Can you work these out from the model? Positions are in its coordinate system, mm. Face numbers are marked on the shaded views. Give positions to 0.01 mm unless a question says otherwise; leave off trailing zeros. Write each loop counter-clockwise with the first axis right and the second up, starting at its lowest first coordinate (ties: lowest second). Pieces come first, ordered by that corner, then holes. Notation, with made-up numbers: (-32, 84.25) -> (-7, 84.25) arc R33 ccw to (-7, 114.25) -> close; hole circle Ø1 at (7.25, -38.5). An arc over 180 degrees is marked (long way). Answer as CSV lines item,"result". Start each with the question number.
1. I need wall thicknesses on line 1 (Y direction, x = 52.5, z = 0.55); line 2 (Y direction, x = -52.5, z = 1.25); line 3 (Y direction, x = 32.5, z = -1.75). Which ranges of each line are inside material? Lowest first, please. Write a range as [from, to].
2. If we section it at D-D on y = -25: Write out the boundary of the cut face in (x, z), plus the area to 3 significant figures.
3. If we section it at B-B on x = 0: Write out the boundary of the cut face in (y, z).
4. I'm going to push flat-ended pins straight in: P1, Ø1.1, axis at x = -16.5, z = -2, coming from the +Y side; P2, Ø9.5, axis at x = -13, y = 5, coming from the +Z side; P3, Ø2, axis at x = -28, z = -2, coming from the -Y side; P4, Ø5, axis at x = -18, y = 22.5, coming from the +Z side. Where does each tip first touch, or does it pass through?
5. If we mould it in two halves opening along Y, with no side actions, what happens to the marked faces 1 and 2? For each: pulls with the +Y half, pulls with the -Y half, needs draft (parallel to the pull), parting line crosses it, or undercut.
6. If we section it at C-C on z = 0.65: Count the separate pieces of the cut face and the enclosed holes in it, plus the area to 3 significant figures.
7. If we section it at A-A on x = -52.5: Write out the boundary of the cut face in (y, z).
```python
from build123d import *

# Parameters (mm, degrees)
SKETCH_1_W          = 113
SKETCH_1_H          = 37
SKETCH_1_R          = 2
EXTRUDE_1_DEPTH     = 2.5
SKETCH_2_W          = 12
SKETCH_2_H          = 15
CUT_EXTRUDE_1_DEPTH = 6
CUT_EXTRUDE_2_DEPTH = 1
FILLET_1_R          = 2
FILLET_2_R          = 2
EXTRUDE_2_DEPTH     = 5
FILLET_3_R          = 10
SKETCH_5_R          = 1.75
CUT_EXTRUDE_3_DEPTH = 6


with BuildPart() as part:
    # 草图1 → 凸台-拉伸1 (new body, symmetric)
    with BuildSketch(Plane.XY):
        Rectangle(SKETCH_1_W, SKETCH_1_H)
        with Locations((52.5, 14.5)):
            Circle(SKETCH_1_R, mode=Mode.SUBTRACT)
        with Locations((52.5, -14.5)):
            Circle(SKETCH_1_R, mode=Mode.SUBTRACT)
        with Locations((-52.5, -14.5)):
            Circle(SKETCH_1_R, mode=Mode.SUBTRACT)
        with Locations((-52.5, 14.5)):
            Circle(SKETCH_1_R, mode=Mode.SUBTRACT)
    extrude(amount=EXTRUDE_1_DEPTH, both=True)

    # 草图2 → 切除-拉伸1 (cut, through all)
    with BuildSketch(Plane(origin=(0, 0, -2.5), x_dir=(-1, 0, 0), z_dir=(0, 0, -1))):
        with Locations((50.5, 0)):
            Rectangle(SKETCH_2_W, SKETCH_2_H)
    extrude(amount=-CUT_EXTRUDE_1_DEPTH, mode=Mode.SUBTRACT)

    # 草图3 → 切除-拉伸2 (cut)
    with BuildSketch(Plane(origin=(0, 0, -2.5), x_dir=(-1, 0, 0), z_dir=(0, 0, -1))):
        Polygon((-48.5, -15.5), (48.500097741, -15.5), (48.500097741, -10.5), (41.5, -10.5), (41.5, 10.420732232), (48.500097741, 10.420732232), (48.526939222, 15.5), (-48.5, 15.5), align=None)
    cut_extrude_2 = extrude(amount=-CUT_EXTRUDE_2_DEPTH, mode=Mode.SUBTRACT)

    # 圆角1
    fillet_1_edges = [part.edges().sort_by_distance(p)[0] for p in [
        (48.5, -15.5, -2),
        (48.5, 15.5, -2),
        (-48.526939222, 15.5, -2),
        (-48.500097741, 10.420732232, -2),
        (-41.5, 10.420732232, -2),
        (-41.5, -10.5, -2),
        (-48.500097741, -10.5, -2),
        (-48.500097741, -15.5, -2),
    ]]
    fillet(fillet_1_edges, radius=FILLET_1_R)

    # 圆角2
    fillet_2_edges = [part.edges().sort_by_distance(p)[0] for p in [
        (-56.5, 7.5, 0),
        (-56.5, -7.5, 0),
        (-44.5, -7.5, 0),
        (-44.5, 7.5, 0),
        (-56.5, 18.5, 0),
        (56.5, 18.5, 0),
        (56.5, -18.5, 0),
        (-56.5, -18.5, 0),
    ]]
    fillet(fillet_2_edges, radius=FILLET_2_R)

    # 草图4 → 凸台-拉伸2 (add)
    with BuildSketch(Plane(origin=(0, 0, -2.5), x_dir=(-1, 0, 0), z_dir=(0, 0, -1))):
        Polygon((17.5, 18.5), (0, 33.5), (-17.5, 18.5), align=None)
        Polygon((17.5, -18.5), (-17.5, -18.5), (0, -33.5), align=None)
    extrude(amount=-EXTRUDE_2_DEPTH)

    # 圆角3
    fillet_3_edges = [part.edges().sort_by_distance(p)[0] for p in [
        (-17.5, 18.5, 0),
        (17.5, 18.5, 0),
        (0, 33.5, 0),
        (0, -33.5, 0),
        (17.5, -18.5, 0),
        (-17.5, -18.5, 0),
    ]]
    fillet(fillet_3_edges, radius=FILLET_3_R)

    # 草图5 → 切除-拉伸3 (cut, through all)
    with BuildSketch(Plane(origin=(0, 0, -2.5), x_dir=(-1, 0, 0), z_dir=(0, 0, -1))):
        with Locations((0, -25)):
            Circle(SKETCH_5_R)
        with Locations((0, 25)):
            Circle(SKETCH_5_R)
    extrude(amount=-CUT_EXTRUDE_3_DEPTH, mode=Mode.SUBTRACT)

    # 镜向1: 切除-拉伸2 across plane
    add(cut_extrude_2.mirror(Plane.XY), mode=Mode.SUBTRACT)


solid = part.part
```
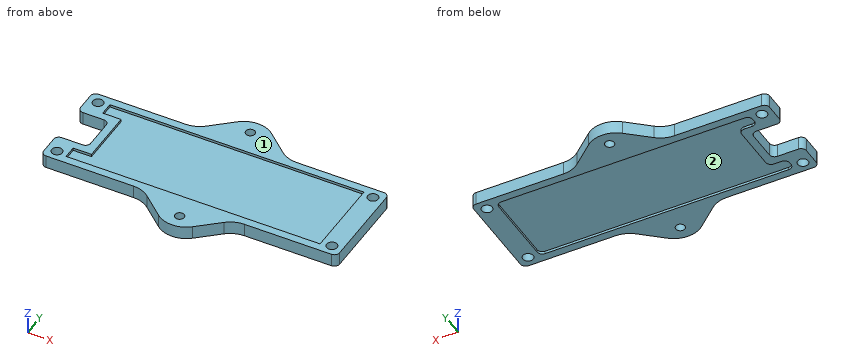
Computed values:
1,line 1,"y = [-18.5, -16.5], [-12.5, 12.5], [16.5, 18.5]"
1,line 2,"y = [-18.5, -16.5], [-12.5, -7.5], [7.5, 12.5], [16.5, 18.5]"
1,line 3,"y = [-18.5, -15.5], [15.5, 18.5]"
2,outline,"(-9.92, -2.5) -> (-1.75, -2.5) -> (-1.75, 2.5) -> (-9.92, 2.5) -> close; (1.75, -2.5) -> (9.92, -2.5) -> (9.92, 2.5) -> (1.75, 2.5) -> close"
2,area,"81.7 mm2"
3,outline,"(-30.33, -2.5) -> (-26.75, -2.5) -> (-26.75, 2.5) -> (-30.33, 2.5) -> close; (-23.25, -2.5) -> (-15.5, -2.5) -> (-15.5, -1.5) -> (15.5, -1.5) -> (15.5, -2.5) -> (23.25, -2.5) -> (23.25, 2.5) -> (15.5, 2.5) -> (15.5, 1.5) -> (-15.5, 1.5) -> (-15.5, 2.5) -> (-23.25, 2.5) -> close; (26.75, -2.5) -> (30.33, -2.5) -> (30.33, 2.5) -> (26.75, 2.5) -> close"
4,P1,"stops at y = 19.99"
4,P2,"stops at z = 1.5"
4,P3,"stops at y = -18.5"
4,P4,"passes through"
5,face 1,"needs draft"
5,face 2,"undercut"
6,separate pieces,"1"
6,enclosed holes,"6"
6,area,"4,430 mm2"
7,outline,"(-18.5, -2.5) -> (-16.5, -2.5) -> (-16.5, 2.5) -> (-18.5, 2.5) -> close; (-12.5, -2.5) -> (-7.5, -2.5) -> (-7.5, 2.5) -> (-12.5, 2.5) -> close; (7.5, -2.5) -> (12.5, -2.5) -> (12.5, 2.5) -> (7.5, 2.5) -> close; (16.5, -2.5) -> (18.5, -2.5) -> (18.5, 2.5) -> (16.5, 2.5) -> close"
